Geometry check sheet. Reference: the model listing, model coordinates, mm. Coordinates: 2 decimals unless noted, no trailing zeros. Write each loop counter-clockwise with the first axis right and the second up, starting at its lowest first coordinate (ties: lowest second). Pieces come first, ordered by that corner, then holes. Notation, with made-up numbers: (51, 53) -> (97, 53) arc R20 cw to (97, 84) -> close; hole circle Ø8 at (-39.75, 54). An arc over 180 degrees is marked (long way). One line per question, with ' | ' between items.
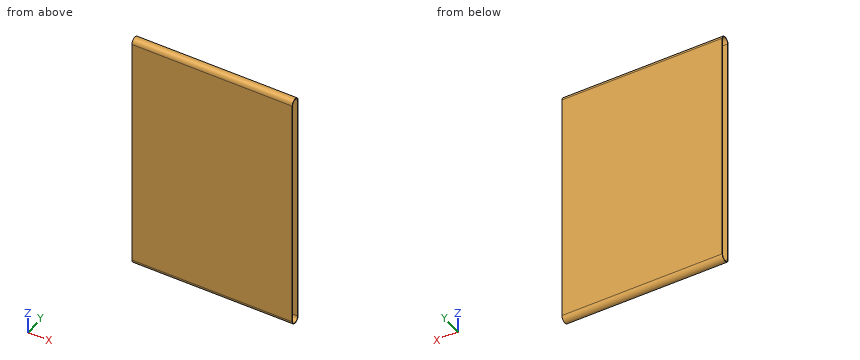
from build123d import *

# Parameters (mm, degrees)
F1_DEPTH = 304.8


with BuildPart() as f1:
    # F0 (on Right) → F1 (new body)
    with BuildSketch(Plane.YZ):
        with BuildLine():
            ThreePointArc((9.2075, 253.882135), (0, 263.089635), (-9.2075, 253.882135))
            Line((-9.2075, 253.882135), (-9.2075, -203.317865))
            ThreePointArc((-9.2075, -203.317865), (0, -212.525365), (9.2075, -203.317865))
            Line((9.2075, -203.317865), (9.2075, 253.882135))
        make_face()
        with BuildLine():
            ThreePointArc((-7.9375, 253.882135), (0, 261.819635), (7.9375, 253.882135))
            Line((7.9375, 253.882135), (7.9375, -203.317865))
            ThreePointArc((7.9375, -203.317865), (0, -211.255365), (-7.9375, -203.317865))
            Line((-7.9375, -203.317865), (-7.9375, 253.882135))
        make_face(mode=Mode.SUBTRACT)
    extrude(amount=F1_DEPTH)


solid = f1.part
1. Go/stop test with a flat-tipped pin: P1, Ø6, axis at x = 206, y = -5, coming from the +Z side. Record where the tip stops, or that it passes through.
Worked answers:
P1: z = 262.87
2. Material ranges on line 1 (Y direction, x = 127.5, z = 48); line 2 (Z direction, x = 268, y = -0.5); line 3 (Z direction, x = 53, y = -7), recorded low to high. Write a range as from..to.
Worked answers:
line 1: -9.21..-7.94, 7.94..9.21 | line 2: -212.51..-211.24, 261.8..263.08 | line 3: -209.3..-207.06, 257.62..259.86
3. Cross-section at B-B on y = 0. Record the boundary of the cut face in (x, z), and give its area (3 significant figures).
Worked answers:
outline: (0, -212.53) -> (304.8, -212.53) -> (304.8, -211.26) -> (0, -211.26) -> close; (0, 261.82) -> (304.8, 261.82) -> (304.8, 263.09) -> (0, 263.09) -> close | area: 774 mm²
4. Cross-section at A-A on z = -107. Record the boundary of the cut face in (x, y).
Worked answers:
outline: (0, -9.21) -> (304.8, -9.21) -> (304.8, -7.94) -> (0, -7.94) -> close; (0, 7.94) -> (304.8, 7.94) -> (304.8, 9.21) -> (0, 9.21) -> close
5. Cross-section at C-C on x = 22.5. Record the boundary of the cut face in (y, z) (1 decimal).
Worked answers:
outline: (-9.2, -203.3) arc R9.2 ccw to (9.2, -203.3) -> (9.2, 253.9) arc R9.2 ccw to (-9.2, 253.9) -> close; hole (-7.9, -203.3) arc R7.9 ccw to (7.9, -203.3) -> (7.9, 253.9) arc R7.9 ccw to (-7.9, 253.9) -> close
